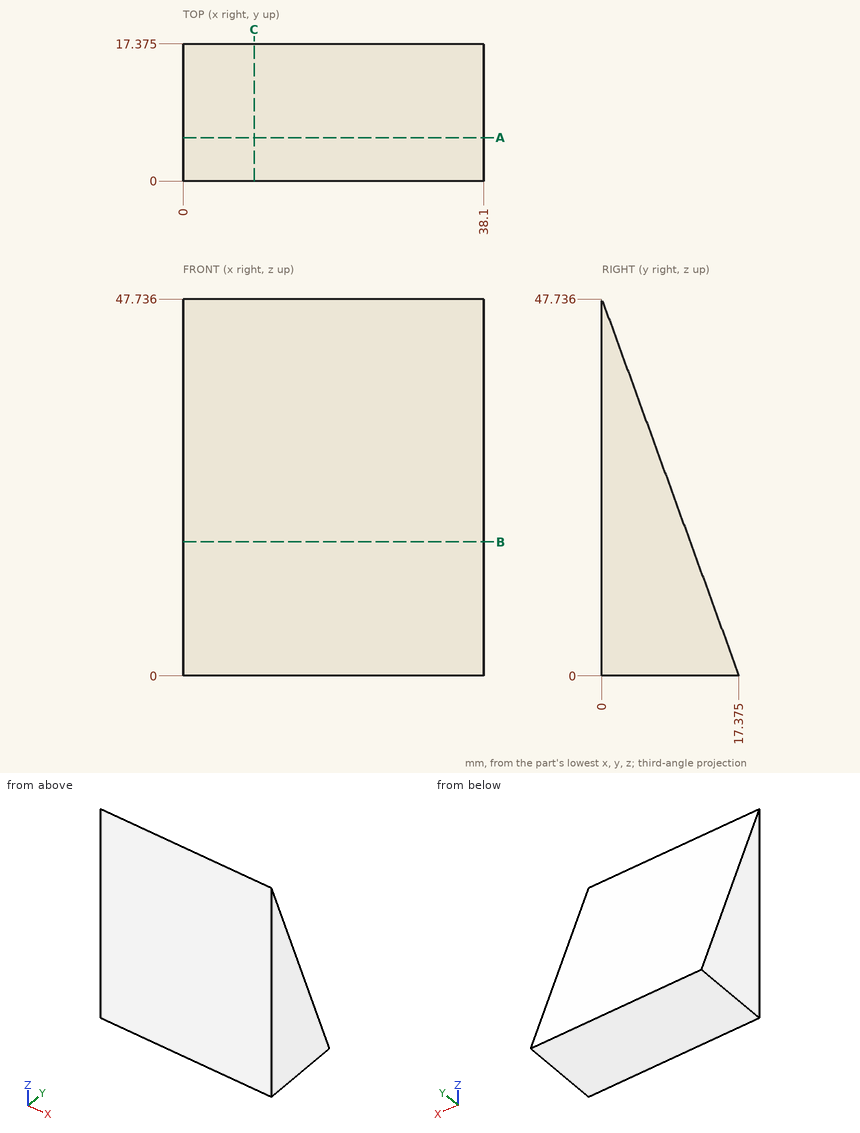
Geometry: see drawing. Coordinates: mm, zero at the bounding-box minimum. Give positions to 0.01 mm unless a question says otherwise; leave off trailing zeros. Loops run counter-clockwise (first coordinate to the right, second up) from the corner with the lowest first, then second, coordinate; pieces in that order, holes last. Notation, with made-up numbers: M 10,-30 L 46,-30 A25 cw 46,0 Z; hole C 58,29.5 d3. An arc over 180 degrees is marked long. Answer as CSV lines item,"result". Start each with the question number.
1. Pin query (flat end, axial travel): P1, Ø4, axis at x = 5, z = 30.5, coming from the +Y side; P2, Ø4, axis at x = 5, z = 34, coming from the +Y side; P3, Ø2, axis at x = 16.5, z = 16, coming from the +Y side (1 decimal). Return the tip coordinate at first contact, or that it passes through.
2. Section B-B on z = 17. Return loops of the section in (x, y).
3. Section A-A on y = 5.5. Return loops of the section in (x, z) (1 decimal), plus the area to 3 significant figures.
4. Section C-C on x = 9. Return loops of the section in (y, z) (1 decimal).
5. Line query: L1, parallel to Y at x = 9, z = 14; L2, parallel to Y at x = 3, z = 37.5 (1 decimal). Output: solid intervals per line, ascending.
Computed values:
1,P1,"stops at y = 7"
1,P2,"stops at y = 5.73"
1,P3,"stops at y = 11.9"
2,outline,"M 0,0 L 38.1,0 L 38.1,11.19 L 0,11.19 Z"
3,outline,"M 0,0 L 38.1,0 L 38.1,32.6 L 0,32.6 Z"
3,area,"1,240 mm²"
4,outline,"M 0,0 L 17.4,0 L 0,47.7 Z"
5,L1,"y = 0 to 12.28"
5,L2,"y = 0 to 3.7"
